Autodesk Inventor part; units mm, degrees
ref_plane "YZ Plane" through (0, 0, 0) normal (1, 0, 0) x (0, 1, 0)
ref_plane "XZ Plane" through (0, 0, 0) normal (0, 1, 0) x (-1, 0, 0)
ref_plane "XY Plane" through (0, 0, 0) normal (0, 0, 1) x (1, 0, 0)
sketch "Sketch1" plane through (0, 0, 0) normal (1, 0, 0) x (0, 1, 0)
  circle A0 centre (0, 0) radius 6.5
  circle A1 centre (0, 0) radius 2
  dimension "d0" = 13
  dimension "d1" = 4
extrude "Extrusion1" add sketch "Sketch1" along normal mid plane 5
fillet "Fillet1" radius 0.25 2 edges at (2.5, -6.5, 0) (-2.5, -6.5, 0)
fillet "Fillet2" radius 0.25 1 edges at (2.5, -2, 0)
sketch "Sketch2" plane through (2.5, 0, 0) normal (1, 0, 0) x (0, 0, -1)
  circle A0 centre (0, 0) radius 5.25
  circle A1 centre (0, 0) radius 4.5
  dimension "d6" = 10.5
  dimension "d7" = 9
extrude "Extrusion2" cut sketch "Sketch2" against normal blind 0.25
mirror "Mirror1" about plane through (0, 0, 0) normal (1, 0, 0) of "Extrusion2"
properties part number "Bearing" material "Stainless Steel, Austenitic"
Geometry check sheet. Reference: the model listing, model coordinates, mm. Give positions to 0.01 mm unless a question says otherwise; leave off trailing zeros. Loops run counter-clockwise (first coordinate to the right, second up) from the corner with the lowest first, then second, coordinate; pieces in that order, holes last. Notation, with made-up numbers: M 59,29 L 83,29 A25 cw 83,68 Z; hole C 58.5,63.5 d4. An arc over 180 degrees is marked long. Answer as a JSON object with one key per item and string values. Group by question number.
Item 1: Mould release check, pull along Z, two halves, no side actions. Record for faces 1 (the cylindrical face through (0, 0, 2)), 2 (the cylindrical face through (-0.031, -5.158, 3.955)), 3 (the flat face through (2.5, 2, -2)): pulls with the +Z half, pulls with the -Z half, needs draft (parallel to the pull), parting line crosses it, or undercut.
Item 2: Gauge pin test, flat ends, axial feed: pin 1 (1.5 mm diameter, centred on x = 0, y = 2.5, fed in from -Z); pin 2 (2.5 mm diameter, centred on y = 0, z = 0, fed in from -X); pin 3 (1.5 mm diameter, centred on x = -0.5, z = 4.5, fed in from -Y); pin 4 (1.5 mm diameter, centred on x = -1.5, z = -5, fed in from -Y). Record the tip position at first contact, or that the pin passes through.
Item 3: Sectioned sample at C-C on x = -1.95. Record the boundary of the cut face in (y, z), plus the area to 3 significant figures.
Item 4: Material ranges on L1, parallel to Z at x = -2.3, y = 3; L2, parallel to X at y = -4.5, z = -0.75; L3, parallel to Z at x = 1.25, y = 0.75, recorded low to high.
Findings below:
{
 "1": {"face 1": "undercut", "face 2": "parting line crosses it", "face 3": "needs draft"},
 "2": {"pin 1": "z = -6.26", "pin 2": "through", "pin 3": "y = -5.31", "pin 4": "y = -4.92"},
 "3": {"outline": "C 0,0 d13; hole C 0,0 d4", "area": "120 mm2"},
 "4": {"L1": "-5.76 to -4.31, -3.35 to 3.35, 4.31 to 5.76", "L2": "-2.25 to 2.25", "L3": "-6.46 to -1.85, 1.85 to 6.46"}
}
